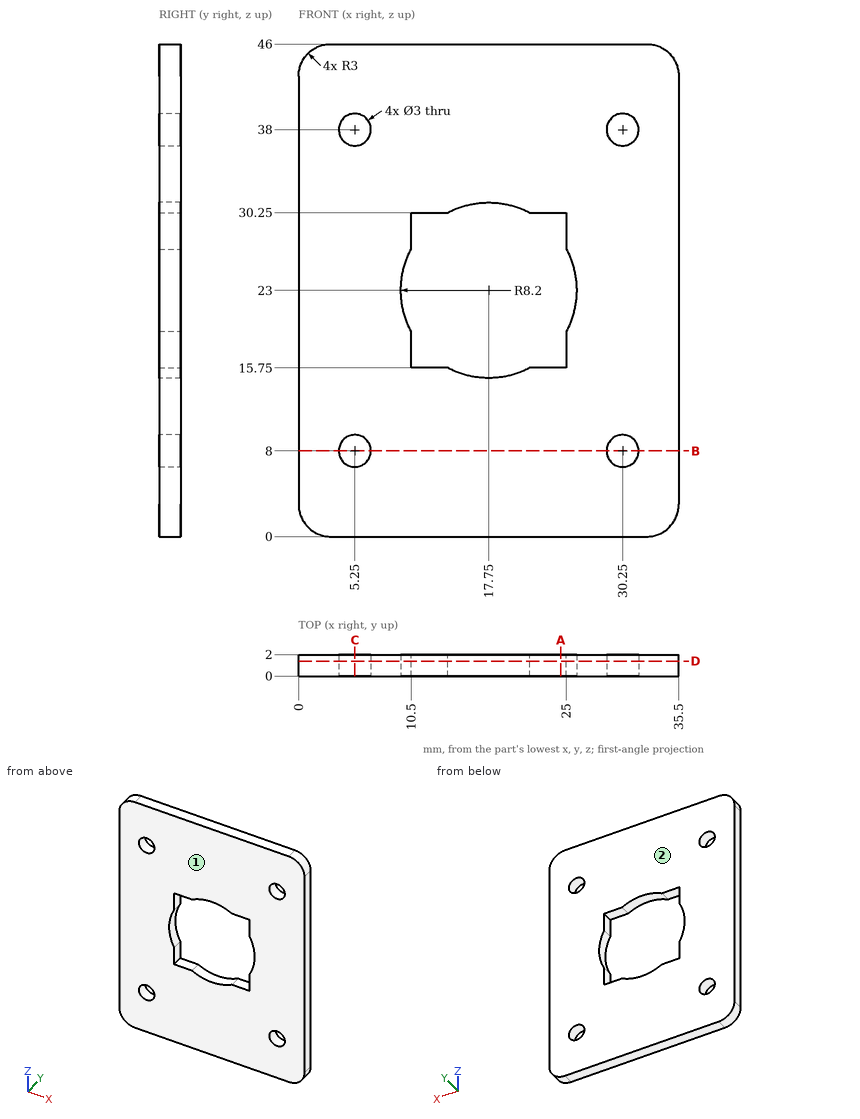
Source: three-view drawing plus pictorial views. Frame: mm from the lowest corner of the part. Coordinates: 2 decimals unless noted, no trailing zeros. Loops run counter-clockwise (first coordinate to the right, second up) from the corner with the lowest first, then second, coordinate; pieces in that order, holes last. Notation, with made-up numbers: (3, -25.5) -> (44, -25.5) arc R13 ccw to (44, -17.5) -> close; hole circle Ø9 at (47.5, 61). An arc over 180 degrees is marked (long way). Write each question's results on one line, items separated by ' | '. Start each with the question number.
Q1. Pin query (flat end, axial travel): pin 1 (2.5 mm diameter, centred on x = 30.25, z = 38, fed in from +Y). Return the tip coordinate at first contact, or that it passes through.
Q2. Section C-C, the plane x = 5.25. Return the cut outline in (y, z), plus the area to 3 significant figures.
Q3. Section B-B, the plane z = 8. Return the cut outline in (x, y), plus the area to 3 significant figures.
Q4. Ray query, line 1 (X direction, y = 1.35, z = 8); line 2 (Z direction, x = 24, y = 0.7); line 3 (Z direction, x = 31.5, y = 1.8). Return the intervals inside material, ascending. Write a range as from..to.
Q5. Section A-A, the plane x = 24.5. Return the cut outline in (y, z).
Q6. Section D-D, the plane y = 1.4. Return the cut outline in (x, z).
Q7. Pull-direction query (Y, two-part tool) for the marked faces 1 and 2; classes: released by +Y, released by -Y, zero draft, split by the parting line, or undercut.
Found:
1) pin 1: through
2) outline: (0, 0) -> (2, 0) -> (2, 6.5) -> (0, 6.5) -> close; (0, 9.5) -> (2, 9.5) -> (2, 36.5) -> (0, 36.5) -> close; (0, 39.5) -> (2, 39.5) -> (2, 46) -> (0, 46) -> close | area: 80.0 mm2
3) outline: (0, 0) -> (3.75, 0) -> (3.75, 2) -> (0, 2) -> close; (6.75, 0) -> (28.75, 0) -> (28.75, 2) -> (6.75, 2) -> close; (31.75, 0) -> (35.5, 0) -> (35.5, 2) -> (31.75, 2) -> close | area: 59.0 mm2
4) line 1: 0..3.75, 6.75..28.75, 31.75..35.5 | line 2: 0..15.75, 30.25..46 | line 3: 0..7.17, 8.83..37.17, 38.83..46
5) outline: (0, 0) -> (2, 0) -> (2, 15.75) -> (0, 15.75) -> close; (0, 30.25) -> (2, 30.25) -> (2, 46) -> (0, 46) -> close
6) outline: (0, 3) arc R3 ccw to (3, 0) -> (32.5, 0) arc R3 ccw to (35.5, 3) -> (35.5, 43) arc R3 ccw to (32.5, 46) -> (3, 46) arc R3 ccw to (0, 43) -> close; hole circle Ø3 at (5.25, 8); hole circle Ø3 at (5.25, 38); hole (10.5, 15.75) -> (13.92, 15.75) arc R8.2 ccw to (21.58, 15.75) -> (25, 15.75) -> (25, 19.17) arc R8.2 ccw to (25, 26.83) -> (25, 30.25) -> (21.58, 30.25) arc R8.2 ccw to (13.92, 30.25) -> (10.5, 30.25) -> (10.5, 26.83) arc R8.2 ccw to (10.5, 19.17) -> close; hole circle Ø3 at (30.25, 8); hole circle Ø3 at (30.25, 38)
7) face 1: released by -Y | face 2: released by +Y
